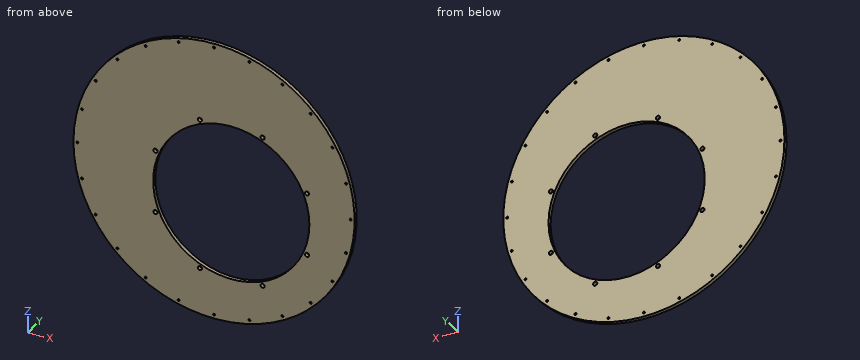
Autodesk Inventor part; units mm, degrees
ref_plane "YZ Plane" through (0, 0, 0) normal (1, 0, 0) x (0, 1, 0)
ref_plane "XZ Plane" through (0, 0, 0) normal (0, 1, 0) x (-1, 0, 0)
ref_plane "XY Plane" through (0, 0, 0) normal (0, 0, 1) x (1, 0, 0)
sketch "Sketch1" plane through (0, 0, 0) normal (0, 1, 0) x (-1, 0, 0)
  circle A0 centre (0, 0) radius 228.6
  dimension "d0" = 457.2
extrude "Extrusion1" add sketch "Sketch1" along normal blind 6.35
sketch "Sketch7" plane through (0, 6.35, 0) normal (0, 1, 0) x (1, 0, 0)
  line L0 (0, 0) -> (0, 222.25)
  dimension "d42" = 222.25
hole "Hole3" at (0, 6.35, -222.25) direction (0, -1, 0) diameter 3.302 end up to surface
pattern_circular "Circular Pattern1" count 24 over 360 about axis through (0, 0, 0) along (0, 1, 0) of "Hole3"
sketch "Sketch8" plane through (0, 6.35, 0) normal (0, 1, 0) x (1, 0, 0)
  line L0 (0, 0) -> (28.0184, 28.0184) construction
  line L1 (0, 0) -> (39.624, 0) construction
  circle A0 centre (28.0184, 28.0184) radius 127
  dimension "d53" = 39.624
  dimension "d54" = 45
  dimension "d55" = 254
extrude "Extrusion4" cut sketch "Sketch8" against normal through all
sketch "Sketch9" plane through (0, 6.35, 0) normal (0, 1, 0) x (1, 0, 0)
  circle A0 centre (28.0184, 28.0184) radius 127
  line L0 (28.0184, 28.0184) -> (151.2177, 79.0492)
  line L1 (28.0184, 28.0184) -> (161.3684, 28.0184) construction
  point P0 (0, 0)
  dimension "d58" = 133.35
  dimension "d59" = 22.5
hole "Hole4" at (151.2177, 6.35, -79.0492) direction (0, -1, 0) diameter 6.7564 end through all
pattern_circular "Circular Pattern2" count 8 over 360 about axis through (28.0184, 6.35, -28.0184) along (0, -1, 0) of "Hole4"
properties part number "55K stage" material "Aluminum 6061"
Can you work these out from the model? Positions are in its coordinate system, mm. Give positions to 0.01 mm unless a question says otherwise; leave off trailing zeros. Write each loop counter-clockwise with the first axis right and the second up, starting at its lowest first coordinate (ties: lowest second). Pieces come first, ordered by that corner, then holes. Notation, with made-up numbers: (62.5, 24.25) -> (88.5, 24.25) arc R31 ccw to (88.5, 62.25) -> close; hole circle Ø11 at (82, 32.5). An arc over 180 degrees is marked (long way). Answer as a JSON object with one key per item and string values. Group by question number.
Item 1: Suppose I cut it at A-A (x = 8). Please give me the cut outline in (y, z), plus the area to 3 significant figures.
Item 2: Please list where these lines run through material, in increasing order: line 1 (Z direction, x = 157.5, y = 1.5); line 2 (X direction, y = 4.25, z = 10); line 3 (X direction, y = 1.25, z = -85.5). Write a range as [from, to].
Item 3: Suppose I cut it at C-C (y = 3.5). State how many separate pieces and enclosed holes the cut face has, plus the area to 3 significant figures.
Item 4: Suppose I cut it at B-B (z = -69.5). Please give me the cut outline in (x, y), plus the area to 3 significant figures.
Item 5: I'm going to push flat-ended pins straight in: P1, Ø5.5, axis at x = 111.12, z = -192.47, coming from the +Y side; P2, Ø2.5, axis at x = 192.47, z = 111.12, coming from the +Y side; P3, Ø3, axis at x = 172.5, y = 5, coming from the +Z side. Where does each tip first touch, or does it pass through?
Findings:
{
 "1": {"outline": "(0, -228.46) -> (6.35, -228.46) -> (6.35, -153.43) -> (0, -153.43) -> close; (0, 97.39) -> (6.35, 97.39) -> (6.35, 228.46) -> (0, 228.46) -> close", "area": "1,310 mm²"},
 "2": {"line 1": "z = [-165.69, -158.77], [-155.54, 155.54], [158.77, 165.69]", "line 2": "x = [-228.38, -93.16], [149.19, 228.38]", "line 3": "x = [-212.01, -85.23], [141.27, 212.01]"},
 "3": {"separate pieces": "1", "enclosed holes": "33", "area": "113,000 mm²"},
 "4": {"outline": "(-217.78, 0) -> (-92.02, 0) -> (-92.02, 6.35) -> (-217.78, 6.35) -> close; (148.05, 0) -> (217.78, 0) -> (217.78, 6.35) -> (148.05, 6.35) -> close", "area": "1,240 mm²"},
 "5": {"P1": "stops at y = 6.35", "P2": "passes through", "P3": "stops at z = 151.71"}
}
